Model file for the job. Use its own axes, mm. Face numbers are marked on the shaded views. Coordinates: 2 decimals unless noted, no trailing zeros. Write each loop counter-clockwise with the first axis right and the second up, starting at its lowest first coordinate (ties: lowest second). Pieces come first, ordered by that corner, then holes. Notation, with made-up numbers: (55.25, 12) - (104.25, 12) arc R19 cw to (104.25, 16) - close; hole circle Ø11 at (63, 54). An arc over 180 degrees is marked (long way). Put each result on its own line as item: value. Start each with the question number.
1. Drop flat-ended pins along their axis: P1, Ø2, axis at x = 3, z = -1, coming from the -Y side; P2, Ø4, axis at x = 0, y = 0, coming from the +Z side. Give the stop position or say it passes through.
2. Saw through at A-A, the plane z = -0.75. Write the cut outline in (x, y) (3 decimals), plus the area to 3 significant figures.
3. Pull direction Y, two halves, no side cores. Call the marked faces 1, 2 and 3: released by +Y, released by -Y, zero draft, split by the parting line, or undercut.
4. Drill centre lines: L1, parallel to X at y = 0, z = 1.4 (3 decimals); L2, parallel to Y at x = 2.5, z = -1.9; L3, parallel to Y at x = 1.5, z = 1.65. Where is each one in solid material? Low to high. Write a range as from..to.
```python
from build123d import *

# Parameters (mm, degrees)
SKETCH1_R               = 3.175
EXTRUDE1_DEPTH          = 2.778125
SKETCH9_OUTSIDE_W       = 55.29
SKETCH9_OUTSIDE_H       = 57.01
SKETCH9_OUTSIDE_R       = 5.55625
CUT_EXTRUDE2_DEPTH      = 11.1442782
CUT_EXTRUDE2_DRAFT      = -60
MIRROR2_COPY_1_SKETCH_W = 55.29
MIRROR2_COPY_1_SKETCH_H = 57.01
MIRROR2_COPY_1_SKETCH_R = 5.55625
MIRROR2_COPY_1_DEPTH    = 11.1442782
MIRROR2_COPY_1_DRAFT    = -60


with BuildPart() as part:
    # Sketch1 → Extrude1 (new, symmetric)
    with BuildSketch(Plane.XY):
        Polygon((-5.55625, 3.207902433), (-5.55625, -3.207902433), (0, -6.415804866), (5.55625, -3.207902433), (5.55625, 3.207902433), (0, 6.415804866), align=None)
        Circle(SKETCH1_R, mode=Mode.SUBTRACT)
    extrude(amount=EXTRUDE1_DEPTH, both=True)


with BuildPart() as cut_extrude2_tool:
    # Sketch9 outside → Cut-Extrude2 (with draft: the straight prism first)
    with BuildSketch(Plane.XY.offset(2.778125)):
        Rectangle(SKETCH9_OUTSIDE_W, SKETCH9_OUTSIDE_H)
        Circle(SKETCH9_OUTSIDE_R, mode=Mode.SUBTRACT)
    extrude(amount=-CUT_EXTRUDE2_DEPTH)
    # Cut-Extrude2: the draft: its side faces are tilted about the plane it starts from
    cut_extrude2_sides = [cut_extrude2_tool.faces().sort_by_distance(p)[0] for p in [
        (0, -28.505, -2.7940141),
        (27.645, 0, -2.7940141),
        (0, 28.505, -2.7940141),
        (-27.645, 0, -2.7940141),
        (-5.55625, 0, -2.7940141),
    ]]
    draft(cut_extrude2_sides, Plane.XY.offset(2.778125), CUT_EXTRUDE2_DRAFT)


with BuildPart() as part_1:
    add(part.part)

    # Cut-Extrude2: cut by cut_extrude2_tool
    add(cut_extrude2_tool.part, mode=Mode.SUBTRACT)


with BuildPart() as mirror2_copy_1_tool:
    # Mirror2 copy 1 sketch → Mirror2 copy 1 (with draft: the straight prism first)
    with BuildSketch(Plane(origin=(0, 0, -2.778125), x_dir=(1, 0, 0), z_dir=(0, 0, -1))):
        Rectangle(MIRROR2_COPY_1_SKETCH_W, MIRROR2_COPY_1_SKETCH_H)
        Circle(MIRROR2_COPY_1_SKETCH_R, mode=Mode.SUBTRACT)
    extrude(amount=-MIRROR2_COPY_1_DEPTH)
    # Mirror2 copy 1: the draft: its side faces are tilted about the plane it starts from
    mirror2_copy_1_sides = [mirror2_copy_1_tool.faces().sort_by_distance(p)[0] for p in [
        (0, -28.505, 2.7940141),
        (27.645, 0, 2.7940141),
        (0, 28.505, 2.7940141),
        (-27.645, 0, 2.7940141),
        (-5.55625, 0, 2.7940141),
    ]]
    draft(mirror2_copy_1_sides, Plane(origin=(0, 0, -2.778125), x_dir=(1, 0, 0), z_dir=(0, 0, -1)), MIRROR2_COPY_1_DRAFT)


with BuildPart() as part_2:
    add(part_1.part)

    # Mirror2 copy 1: cut by mirror2_copy_1_tool
    add(mirror2_copy_1_tool.part, mode=Mode.SUBTRACT)

    # Cut-Extrude10 cone 1 section (through the dimple's axis) → Cut-Extrude10 (revolve, cut)
    with BuildSketch(Plane(origin=(0, 0, 2.778125), x_dir=(0, -1, 0), z_dir=(1, 0, 0))):
        Polygon((0, 0), (3.429, 0), (0, 3.429), align=None)
    revolve(axis=Axis((0, 0, 2.778125), (0, 0, -1)), mode=Mode.SUBTRACT)


solid = part_2.part
```
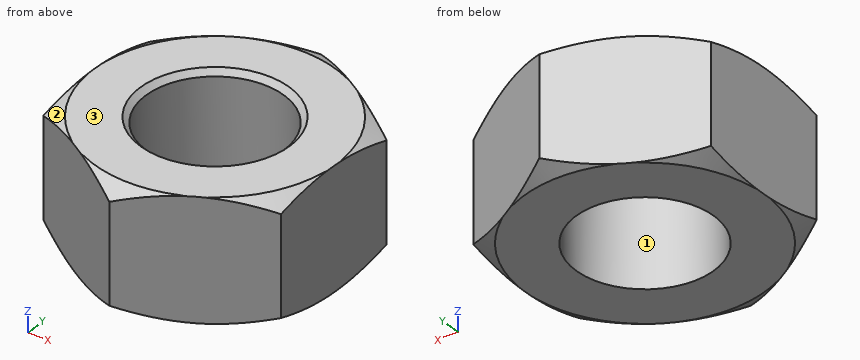
Final values:
1. P1: stops at y = -5.26
1. P2: passes through
2. outline: (-5.556, -3.208) - (0, -6.416) - (5.556, -3.208) - (5.556, 3.208) - (0, 6.416) - (-5.556, 3.208) - close; hole circle Ø6.35 at (0, 0)
2. area: 75.3 mm²
3. face 1: undercut
3. face 2: released by -Y
3. face 3: zero draft
4. L1: x = -5.556..-3.175, 3.175..5.556
4. L2: y = -4.97..-1.96, 1.96..4.97
4. L3: y = -5.55..-2.8, 2.8..5.55
